Input: part model. Units: mm. Frame: model coordinates. Face numbers are marked on the shaded views. A direction names the side the tool comes from. Coordinates: 2 decimals unless noted, no trailing zeros. Loops run counter-clockwise (first coordinate to the right, second up) from the corner with the lowest first, then second, coordinate; pieces in that order, holes last.
```python
from build123d import *

# Parameters (mm, degrees)
SKETCH1_W                    = 20
SKETCH1_H                    = 20
BASE_FLANGE1_DEPTH           = 0.9
EDGE_FLANGE2_DEPTH           = 20
F_25_0_1495_DIAMETER_SLOT2_D = 3.7973
EDGE_FLANGE4_DEPTH           = 20
F_25_0_1495_DIAMETER_SLOT5_D = 3.7973


# Sheet-metal steps are written as plain solids
with BuildPart() as part:
    # Sketch1 → Base-Flange1 (new body)
    with BuildSketch(Plane.XY):
        Rectangle(SKETCH1_W, SKETCH1_H)
    extrude(amount=-BASE_FLANGE1_DEPTH)

    # Edge-Flange2 section (across the edge) → Edge-Flange2 (add)
    with BuildSketch(Plane(origin=(-10, 11, -0.9), x_dir=(0, -1, 0), z_dir=(1, 0, 0))):
        with BuildLine():
            Line((-0.9, 1), (-0.9, 27))
            Line((-0.9, 27), (0, 27))
            Line((0, 27), (0, 1))
            ThreePointArc((0, 1), (0.292893219, 0.292893219), (1, 0))
            Line((1, 0), (1, -0.9))
            ThreePointArc((1, -0.9), (-0.343502884, -0.343502884), (-0.9, 1))
        make_face()
    extrude(amount=EDGE_FLANGE2_DEPTH)

    # #25 (0.1495) Diameter Slot2 (through all)
    with Locations(Plane(origin=(0, 11.9, 0), x_dir=(1, 0, 0), z_dir=(0, 1, 0))):
        with Locations((0, 17.9)):
            Hole(F_25_0_1495_DIAMETER_SLOT2_D / 2)

    # Edge-Flange4 section (across the edge) → Edge-Flange4 (add)
    with BuildSketch(Plane(origin=(11, -10, 0), x_dir=(-1, 0, 0), z_dir=(0, 1, 0))):
        with BuildLine():
            Line((-0.9, 1), (-0.9, 25))
            Line((-0.9, 25), (0, 25))
            Line((0, 25), (0, 1))
            ThreePointArc((0, 1), (0.292893219, 0.292893219), (1, 0))
            Line((1, 0), (1, -0.9))
            ThreePointArc((1, -0.9), (-0.343502884, -0.343502884), (-0.9, 1))
        make_face()
    extrude(amount=EDGE_FLANGE4_DEPTH)

    # #25 (0.1495) Diameter Slot5 (through all)
    with Locations(Plane.ZY.offset(-11)):
        with Locations((14, 0)):
            Hole(F_25_0_1495_DIAMETER_SLOT5_D / 2)


solid = part.part
```
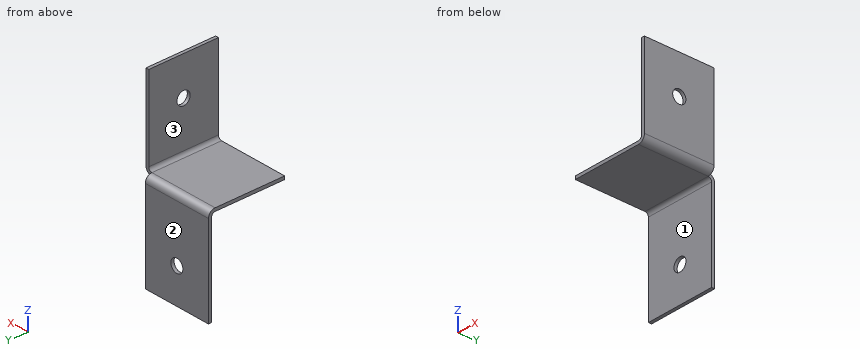
Item 1: Contact query for flat-ended pins moving along their axis: P1, Ø6, axis at x = -7, y = -2, coming from the -Z side; P2, Ø0.6, axis at x = 11, z = 10, coming from the +Y side; P3, Ø1.5, axis at y = 11, z = -16, coming from the +X side; P4, Ø8, axis at x = 2, z = -3.5, coming from the -Y side. Output: stop coordinate, or through.
Result:
P1: stops at z = -0.9
P2: stops at y = 10
P3: stops at x = 10
P4: stops at y = -10
Item 2: Section query A-A (x = 0). Output: boundary loops of the cut face in (y, z), then the cut area to 3 significant figures.
Result:
outline: (-10, -0.9) - (10, -0.9) arc R1 cw to (11, -1.9) - (11, -16) - (11.9, -16) - (11.9, -1.9) arc R1.9 ccw to (10, 0) - (-10, 0) - close; (11, -27.9) - (11.9, -27.9) - (11.9, -19.8) - (11, -19.8) - close
area: 40.0 mm2
Item 3: Reachability of the marked faces 1, 2 and 3 from +Z, -Z, +X, -X, +Y, -Y: full face, straight path, thin tool, end or side. Return the list, or none.
Result:
face 1: -Z, +X, -X, -Y
face 2: +Z, -Z, +X, -X, +Y
face 3: +Z, -X, +Y, -Y
Item 4: Section query D-D (y = 6). Output: boundary loops of the cut face in (x, z).
Result:
outline: (-10, -0.9) - (10, -0.9) arc R1.9 ccw to (11.9, 1) - (11.9, 25) - (11, 25) - (11, 1) arc R1 cw to (10, 0) - (-10, 0) - close
Item 5: Section query C-C (y = 0). Output: boundary loops of the cut face in (x, z).
Result:
outline: (-10, -0.9) - (10, -0.9) arc R1.9 ccw to (11.9, 1) - (11.9, 12.1) - (11, 12.1) - (11, 1) arc R1 cw to (10, 0) - (-10, 0) - close; (11, 15.9) - (11.9, 15.9) - (11.9, 25) - (11, 25) - close
Item 6: Line query: L1, parallel to X at y = 11.35, z = -17.9; L2, parallel to Y at x = 7, z = -17. Output: solid intervals per line, ascending.
Result:
L1: x = -10 to -1.9, 1.9 to 10
L2: y = 11 to 11.9
Item 7: Section query B-B (z = -17.9). Output: boundary loops of the cut face in (x, y).
Result:
outline: (-10, 11) - (-1.9, 11) - (-1.9, 11.9) - (-10, 11.9) - close; (1.9, 11) - (10, 11) - (10, 11.9) - (1.9, 11.9) - close
